Geometry: final body of the model. Coordinates: model frame, mm. A direction names the side the tool comes from. Coordinates: 2 decimals unless noted, no trailing zeros. Order: outer loops, then holes, each group sorted by start corner. A loop starts at its lowest first (then second) coordinate and runs counter-clockwise, first axis right, second up. Notation, with made-up numbers: M 42,61 L 57,61 A22 cw 57,75 Z; hole C -37,65 d2. An arc over 180 degrees is marked long. Write item = value, one per line.
from build123d import *

# Parameters (mm, degrees)
BOSS_EXTRUDE1_DEPTH     = 7.5
CHAMFER1_SIZE           = 1
SKETCH2_R               = 1.8
CUT_EXTRUDE1_DEPTH      = 3
CUT_EXTRUDE1_DEPTH_BACK = 3
FILLET1_R               = 1.5
CHAMFER2_SIZE           = 1.5


with BuildPart() as part:
    # Sketch1 → Boss-Extrude1 (new body, symmetric)
    with BuildSketch(Plane(origin=(0, 0, 0), x_dir=(0, 0, -1), z_dir=(1, 0, 0))):
        Polygon((-5.25, -4.15), (-5.25, -6.15), (6.75, -6.15), (6.75, 6.15), (2.25, 6.15), (2.25, 4.15), (5.25, 4.15), (5.25, 1.85), (0.25, 1.85), (0.25, -0.15), (5.25, -0.15), (5.25, -4.15), align=None)
    extrude(amount=BOSS_EXTRUDE1_DEPTH, both=True)

    # Chamfer1
    chamfer1_edges = [part.edges().sort_by_distance(p)[0] for p in [
        (0, -4.15, -5.25),
        (0, -0.15, -5.25),
    ]]
    chamfer(chamfer1_edges, length=CHAMFER1_SIZE)

    # Sketch2 → Cut-Extrude1 (cut, two sides)
    with BuildSketch(Plane(origin=(0, -4.15, 0), x_dir=(1, 0, 0), z_dir=(0, 1, 0))) as cut_extrude1_sk:
        with Locations((-3.7, -1.15)):
            Circle(SKETCH2_R)
        with Locations((3.7, -1.15)):
            Circle(SKETCH2_R)
    extrude(amount=CUT_EXTRUDE1_DEPTH, mode=Mode.SUBTRACT)
    extrude(cut_extrude1_sk.sketch, amount=-CUT_EXTRUDE1_DEPTH_BACK, mode=Mode.SUBTRACT)

    # Fillet1
    fillet1_edges = [part.edges().sort_by_distance(p)[0] for p in [
        (0, 6.15, -6.75),
        (0, -6.15, -6.75),
    ]]
    fillet(fillet1_edges, radius=FILLET1_R)

    # Chamfer2
    chamfer2_edges = [part.edges().sort_by_distance(p)[0] for p in [
        (0, 4.15, -2.25),
        (0, -0.15, -0.25),
    ]]
    chamfer(chamfer2_edges, length=CHAMFER2_SIZE)


solid = part.part
1) Section D-D, the plane y = 2.75. Return loops of the section in (x, z), and give its area (3 significant figures).
Numbers:
outline = M -7.5,-6.75 L 7.5,-6.75 L 7.5,-5.25 L -7.5,-5.25 Z
area = 22.5 mm²
2) Pin query (flat end, axial travel): pin 1 (4.5 mm diameter, centred on x = 3.7, z = 1.15, fed in from +Y); pin 2 (4 mm diameter, centred on x = -4, z = -5.5, fed in from -Y); pin 3 (2 mm diameter, centred on x = -0.5, y = -2.5, fed in from +Z); pin 4 (5 mm diameter, centred on x = 5, y = 4, fed in from +Z). Return the tip coordinate at first contact, or that it passes through.
Numbers:
pin_1 = 1.85
pin_2 = -6.15
pin_3 = -4.9
pin_4 = -0.25
3) Set-up query: faces 1 (the face through (0, 0, -6.75)), 2 (the face through (0, 4.15, -4)), 3 (the face through (1.9, -5.1, 1.1)). Return all of +Z, -Z, +X, -X, +Y, -Y with unobstructed straight access to the full face (end or side cutting, diameter ignored); none if empty.
Numbers:
face_1 = -Z, +X, -X, +Y, -Y
face_2 = +Z, +X, -X
face_3 = -Y
4) Mould query, pull axis Z, two halves, no side actions, for faces 4 (the face through (-0.1, 4.9, -3)), 5 (the face through (0.11, -5.72, -6.3)), 6 (the face through (-7.5, 0.03, -2.94)), 7 (the face through (-1.983, -5.136, 0.609)). Classes: pulls with the +Z half, pulls with the -Z half, needs draft (parallel to the pull), parting line crosses it, or undercut.
Numbers:
face_4 = pulls with the +Z half
face_5 = pulls with the -Z half
face_6 = needs draft
face_7 = undercut
5) Line query: L1, parallel to X at y = -4.65, z = 1.15; L2, parallel to Y at x = -3.75, z = -4; L3, parallel to Y at x = 4, z = -4.75. Output: solid intervals per line, ascending.
Numbers:
L1 = -7.5 to -5.5, -1.9 to 1.9, 5.5 to 7.5
L2 = -6.15 to -4.15, -0.15 to 1.85, 4.15 to 6.15
L3 = -6.15 to -3.65, -0.65 to 1.85, 4.15 to 6.15
6) Section C-C, the plane x = 6.25. Return loops of the section in (y, z), and give its area (3 significant figures).
Numbers:
outline = M -6.15,-5.25 A1.5 ccw -4.65,-6.75 L 4.65,-6.75 A1.5 ccw 6.15,-5.25 L 6.15,-2.25 L 5.65,-2.25 L 4.15,-3.75 L 4.15,-5.25 L 1.85,-5.25 L 1.85,-0.25 L 1.35,-0.25 L -0.15,-1.75 L -0.15,-4.25 L -1.15,-5.25 L -3.15,-5.25 L -4.15,-4.25 L -4.15,5.25 L -6.15,5.25 Z
area = 53.2 mm²
7) Section B-B, the plane z = 1.15. Return loops of the section in (x, y), and give its area (3 significant figures).
Numbers:
outline = M -7.5,-6.15 L -5.5,-6.15 L -5.5,-4.15 L -7.5,-4.15 Z; M -1.9,-6.15 L 1.9,-6.15 L 1.9,-4.15 L -1.9,-4.15 Z; M 5.5,-6.15 L 7.5,-6.15 L 7.5,-4.15 L 5.5,-4.15 Z
area = 15.6 mm²
8) Section A-A, the plane x = -3.7. Return loops of the section in (y, z).
Numbers:
outline = M -6.15,-5.25 A1.5 ccw -4.65,-6.75 L 4.65,-6.75 A1.5 ccw 6.15,-5.25 L 6.15,-2.25 L 5.65,-2.25 L 4.15,-3.75 L 4.15,-5.25 L 1.85,-5.25 L 1.85,-0.25 L 1.35,-0.25 L -0.15,-1.75 L -0.15,-4.25 L -1.15,-5.25 L -3.15,-5.25 L -4.15,-4.25 L -4.15,-0.65 L -6.15,-0.65 Z; M -6.15,2.95 L -4.15,2.95 L -4.15,5.25 L -6.15,5.25 Z
